Model file for the job. Use its own axes, mm. A direction names the side the tool comes from. Round coordinates to 2 decimals unless told otherwise and drop trailing zeros. Order: outer loops, then holes, each group sorted by start corner. A loop starts at its lowest first (then second) coordinate and runs counter-clockwise, first axis right, second up. Notation, with made-up numbers: (43, -19.5) -> (53, -19.5) arc R29 cw to (53, 11.5) -> close; hole circle Ø7 at (-23, 1.25). An arc over 180 degrees is marked (long way). Use CSV: the item, a comma, the result in double quotes.
```python
from build123d import *

# Parameters (mm, degrees)
BOX005009014_W         = 30
BOX005009014_H         = 5
BOX005009014_DEPTH     = 5
CHAMFER016_SIZE        = 4
CHAMFER017_SIZE        = 4
CHAMFER019_SIZE        = 3.9
BOX005009012_W         = 19.5
BOX005009012_H         = 400
BOX005009012_DEPTH     = 8
CYLINDER023_R          = 3.1
CYLINDER023_DEPTH      = 6
CYLINDER023_ROLL_ANGLE = 90
CHAMFER011_SIZE        = 2.9
CHAMFER009_SIZE        = 2.9
CYLINDER018_R          = 18.5
CYLINDER018_DEPTH      = 3
CYLINDER018_ROLL_ANGLE = 90
CYLINDER017_R          = 16.5
CYLINDER017_DEPTH      = 10
CYLINDER017_ROLL_ANGLE = 90
CYLINDER016_R          = 18.5
CYLINDER016_DEPTH      = 3
CYLINDER016_ROLL_ANGLE = 90
CHAMFER023_SIZE        = 1.9
CHAMFER024_SIZE        = 1.9
CHAMFER025_SIZE        = 1.9


with BuildPart() as chamfer019:
    # Box005009014 → Box005009014 (new body)
    with BuildSketch(Plane(origin=(-7, 261, 13), x_dir=(1, 0, 0), z_dir=(0, 0, 1))):
        with Locations((15, 2.5)):
            Rectangle(BOX005009014_W, BOX005009014_H)
    extrude(amount=BOX005009014_DEPTH)

    # Chamfer016
    chamfer016_edges = [chamfer019.edges().sort_by_distance(p)[0] for p in [
        (-7, 263.5, 18),
    ]]
    chamfer(chamfer016_edges, length=CHAMFER016_SIZE)

    # Chamfer017
    chamfer017_edges = [chamfer019.edges().sort_by_distance(p)[0] for p in [
        (23, 263.5, 18),
    ]]
    chamfer(chamfer017_edges, length=CHAMFER017_SIZE)

    # Chamfer019
    chamfer019_edges = [chamfer019.edges().sort_by_distance(p)[0] for p in [
        (8, 266, 18),
    ]]
    chamfer(chamfer019_edges, length=CHAMFER019_SIZE)


with BuildPart() as part_mirroring005:
    # Part__Mirroring005: instance of Chamfer019
    add(chamfer019.part.mirror(Plane(origin=(0, 250, 0), x_dir=(1, 0, 0), z_dir=(0, 1, 0))))


with BuildPart() as part_mirroring005_1:
    # Part__Mirroring005 placement: moved
    add(part_mirroring005.part.moved(Location((0, 86, 0))))


with BuildPart() as scale_hole001:
    # Box005009012 → Box005009012 (new body)
    with BuildSketch(Plane(origin=(-2, 0, -2), x_dir=(1, 0, 0), z_dir=(0, 0, 1))):
        with Locations((9.75, 200)):
            Rectangle(BOX005009012_W, BOX005009012_H)
    extrude(amount=BOX005009012_DEPTH)


with BuildPart() as lug_hole:
    # Cylinder023 → Cylinder023 (new body)
    with BuildSketch(Plane.XY):
        Circle(CYLINDER023_R)
    extrude(amount=CYLINDER023_DEPTH)


with BuildPart() as lug_hole_1:
    # Cylinder023 roll: moved
    add(lug_hole.part.rotate(Axis((0, 0, 0), (1, 0, 0)), CYLINDER023_ROLL_ANGLE))


with BuildPart() as lug_hole_2:
    # Cylinder023 placement: moved
    add(lug_hole_1.part.moved(Location((7.75, 328, -7))))


with BuildPart() as chamfer011:
    # Chamfer011 base: copy of lug-hole
    add(lug_hole_2.part)

    # Chamfer011
    chamfer011_edges = [chamfer011.edges().sort_by_distance(p)[0] for p in [
        (4.65, 328, -7),
    ]]
    chamfer(chamfer011_edges, length=CHAMFER011_SIZE)


with BuildPart() as chamfer011_1:
    # Chamfer011 placement: moved
    add(chamfer011.part.moved(Location((6, 0, 0))))


with BuildPart() as lug_holes:
    # Chamfer009 base: copy of lug-hole
    add(lug_hole_2.part)

    # Chamfer009
    chamfer009_edges = [lug_holes.edges().sort_by_distance(p)[0] for p in [
        (4.65, 328, -7),
    ]]
    chamfer(chamfer009_edges, length=CHAMFER009_SIZE)


with BuildPart() as lug_holes_1:
    # Chamfer009 placement: moved
    add(lug_holes.part.moved(Location((-6, 0, 0))))

    # Fusion013: union Chamfer011
    add(chamfer011_1.part)


with BuildPart() as end_cheek001:
    # Cylinder018 → Cylinder018 (new body)
    with BuildSketch(Plane.XY):
        Circle(CYLINDER018_R)
    extrude(amount=CYLINDER018_DEPTH)


with BuildPart() as end_cheek001_1:
    # Cylinder018 roll: moved
    add(end_cheek001.part.rotate(Axis((0, 0, 0), (1, 0, 0)), CYLINDER018_ROLL_ANGLE))


with BuildPart() as end_cheek001_2:
    # Cylinder018 placement: moved
    add(end_cheek001_1.part.moved(Location((7.75, 486, 2))))


with BuildPart() as cable_tie_cyl001:
    # Cylinder017 → Cylinder017 (new body)
    with BuildSketch(Plane.XY):
        Circle(CYLINDER017_R)
    extrude(amount=CYLINDER017_DEPTH)


with BuildPart() as cable_tie_cyl001_1:
    # Cylinder017 roll: moved
    add(cable_tie_cyl001.part.rotate(Axis((0, 0, 0), (1, 0, 0)), CYLINDER017_ROLL_ANGLE))


with BuildPart() as cable_tie_cyl001_2:
    # Cylinder017 placement: moved
    add(cable_tie_cyl001_1.part.moved(Location((7.75, 485, 2))))


with BuildPart() as slider_end_l:
    # Cylinder016 → Cylinder016 (new body)
    with BuildSketch(Plane.XY):
        Circle(CYLINDER016_R)
    extrude(amount=CYLINDER016_DEPTH)


with BuildPart() as slider_end_l_1:
    # Cylinder016 roll: moved
    add(slider_end_l.part.rotate(Axis((0, 0, 0), (1, 0, 0)), CYLINDER016_ROLL_ANGLE))


with BuildPart() as slider_end_l_2:
    # Cylinder016 placement: moved
    add(slider_end_l_1.part.moved(Location((7.75, 477, 2))))

    # Fusion010: union end-cheek001, cable-tie-cyl001
    add(end_cheek001_2.part)
    add(cable_tie_cyl001_2.part)


with BuildPart() as slider_end_l_3:
    # Fusion010 placement: moved
    add(slider_end_l_2.part.moved(Location((0, -149, 0))))

    # Cut016: cut lug-holes
    add(lug_holes_1.part, mode=Mode.SUBTRACT)

    # Cut019: cut scale-hole001
    add(scale_hole001.part, mode=Mode.SUBTRACT)

    # Fusion021: union Part__Mirroring005
    add(part_mirroring005_1.part)

    # Chamfer023
    chamfer023_edges = [slider_end_l_3.edges().sort_by_distance(p)[0] for p in [
        (-8.75, 328, 2),
    ]]
    chamfer(chamfer023_edges, length=CHAMFER023_SIZE)

    # Chamfer024
    chamfer024_edges = [slider_end_l_3.edges().sort_by_distance(p)[0] for p in [
        (-10.75, 337, 2),
    ]]
    chamfer(chamfer024_edges, length=CHAMFER024_SIZE)

    # Chamfer025
    chamfer025_edges = [slider_end_l_3.edges().sort_by_distance(p)[0] for p in [
        (-8.75, 334, 2),
    ]]
    chamfer(chamfer025_edges, length=CHAMFER025_SIZE)


solid = slider_end_l_3.part
```
Q1. Pin check, flat tips, straight feed: pin 1 (4 mm diameter, centred on y = 331.5, z = 4, fed in from -X); pin 2 (1.5 mm diameter, centred on x = 18, y = 331.5, fed in from +Z); pin 3 (9 mm diameter, centred on x = 7, z = 3.5, fed in from -Y). Stop position of each tip, or through.
From the geometry:
pin 1,"stops at x = -10.05"
pin 2,"stops at z = 15.49"
pin 3,"stops at y = 325"
Q2. Cut at A-A (x = 7.75). Give the cut face in (y, z), plus the area to 3 significant figures.
From the geometry:
outline,"(320, 13) -> (325, 13) -> (325, 6) -> (337, 6) -> (337, 18.6) -> (335.1, 20.5) -> (334, 20.5) -> (334, 20.4) -> (332.1, 18.5) -> (329.9, 18.5) -> (328, 20.4) -> (328, 20.5) -> (325, 20.5) -> (325, 18) -> (323.9, 18) -> (320, 14.1) -> close; (325, -16.5) -> (328, -16.5) -> (328, -16.4) -> (329.9, -14.5) -> (332.1, -14.5) -> (334, -16.4) -> (334, -16.5) -> (335.1, -16.5) -> (337, -14.6) -> (337, -2) -> (325, -2) -> close"
area,"345 mm²"
Q3. Cut at B-B (y = 323). Give the cut face in (x, z), plus the area to 3 significant figures.
From the geometry:
outline,"(-7, 13) -> (23, 13) -> (23, 14) -> (19.9, 17.1) -> (-3.9, 17.1) -> (-7, 14) -> close"
area,"113 mm²"
Q4. Probe line 1 along X through (y, z) = (325.15, -7); line 2 along Z through (x, y) = (13.75, 325.1); line 3 along Z through (x, y) = (1.75, 325.15). List the from-to ranges inside material, lowest first.
From the geometry:
line 1,"x = -8.41 to -1.3, 4.8 to 10.7, 16.8 to 23.91"
line 2,"z = -15.5 to -10.1, -3.9 to -2, 6 to 19.5"
line 3,"z = -15.5 to -10.05, -3.95 to -2, 6 to 19.5"
Q5. Mould opens along Z. For faces 5 (the flat face through (7.8, 320, 13.5)), 6 (the flat face through (7.8, 324.4, 18)), 7 (the flat face through (8, 322, 13)), 8 (the conical face through (13.224, 327.537, -7.403)) say: +Z half, -Z half, draft (parallel to the pull), parting line (faces both ways), or undercut.
From the geometry:
face 5,"draft"
face 6,"+Z half"
face 7,"-Z half"
face 8,"undercut"
Q6. Which spindle directions (+Z, -Z, +X, -X, +Y, -Y) get a long thin tool onto all of the face, cutting with end or side? Do faces 1 (the flat face through (8, 337, -5)), 2 (the flat face through (-4.5, 325, 16.1)), 3 (the flat face through (8, 331, -2)), 4 (the cylindrical face through (-6.9, 334.6, -9.3)). Say none if no direction does.
From the geometry:
face 1,"+Z, -Z, +X, -X, +Y"
face 2,"+Z, -X, +Y"
face 3,"+Y, -Y"
face 4,"+Y"
